Can you work these out from the model? Positions are in its coordinate system, mm. Face numbers are marked on the shaded views. A direction names the side the tool comes from. Coordinates: 2 decimals unless noted, no trailing zeros. Loops run counter-clockwise (first coordinate to the right, second up) from the corner with the lowest first, then second, coordinate; pieces in that order, holes last.
```python
from build123d import *

# Parameters (mm, degrees)
PAD_DEPTH    = 10
SKETCH001_W  = 20
SKETCH001_H  = 50
PAD001_DEPTH = 10
SKETCH002_W  = 20
SKETCH002_H  = 30
PAD002_DEPTH = 20
SKETCH003_W  = 40
SKETCH003_H  = 20
PAD003_DEPTH = 20


with BuildPart() as part:
    # Sketch → Pad (new body)
    with BuildSketch(Plane.XY):
        Polygon((-45, 50), (-45, 0), (15, 0), (15, 20), (45, 20), (45, 50), align=None)
    extrude(amount=PAD_DEPTH)

    # Sketch001 → Pad001 (new body)
    with BuildSketch(Plane.XY.offset(10)):
        with Locations((-35, 25)):
            Rectangle(SKETCH001_W, SKETCH001_H)
    extrude(amount=PAD001_DEPTH)

    # Sketch002 → Pad002 (new body)
    with BuildSketch(Plane.XY.offset(20)):
        with Locations((-35, 35)):
            Rectangle(SKETCH002_W, SKETCH002_H)
    extrude(amount=PAD002_DEPTH)

    # Sketch003 → Pad003 (new body)
    with BuildSketch(Plane.XY.offset(10)):
        with Locations((-5, 40)):
            Rectangle(SKETCH003_W, SKETCH003_H)
    extrude(amount=PAD003_DEPTH)


solid = part.part
```
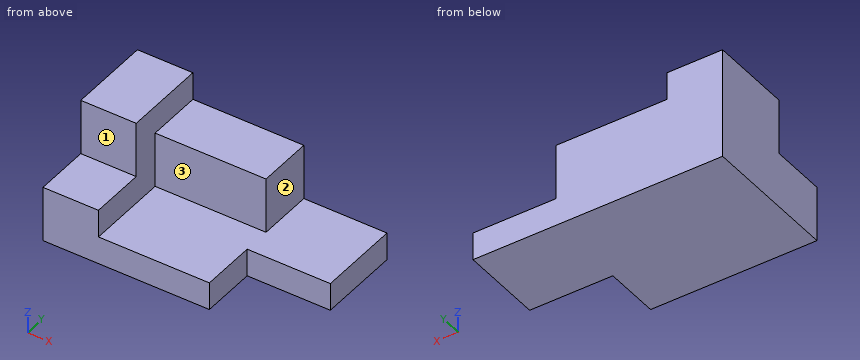
Item 1: On a 3-axis mill with a long thin cutter (end or side, diameter ignored), from which of +Z, -Z, +X, -X, +Y, -Y can I reach the whole of each face in a straight line? I mean the marked faces 1, 2 and 3. Say none if no direction works.
Results are:
face 1: +Z, +X, -X, -Y
face 2: +Z, +X, +Y, -Y
face 3: +Z, +X, -Y
Item 2: Suppose I cut it at D-D, the plane y = 37.5. Please give me the cut outline in (x, z), plus the area to 3 significant figures.
Results are:
outline: (-45, 0) - (45, 0) - (45, 10) - (15, 10) - (15, 30) - (-25, 30) - (-25, 40) - (-45, 40) - close
area: 2,300 mm2
Item 3: Suppose I cut it at B-B, the plane y = 24. Please give me the cut outline in (x, z), plus the area to 3 significant figures.
Results are:
outline: (-45, 0) - (45, 0) - (45, 10) - (-25, 10) - (-25, 40) - (-45, 40) - close
area: 1,500 mm2
Item 4: I'm going to push flat-ended pins straight in: P1, Ø5, axis at x = 7.5, y = 25.5, coming from the +Z side; P2, Ø6, axis at y = 14, z = 24.5, coming from the -X side; P3, Ø15, axis at x = 8.5, y = 37, coming from the +Z side; P4, Ø2, axis at y = 29.5, z = 33.5, coming from the +X side. Where does each tip first touch, or does it pass through?
Results are:
P1: stops at z = 10
P2: passes through
P3: stops at z = 30
P4: stops at x = -25
Item 5: Suppose I cut it at A-A, the plane z = 13. Please give me the cut outline in (x, y), plus the area to 3 significant figures.
Results are:
outline: (-45, 0) - (-25, 0) - (-25, 30) - (15, 30) - (15, 50) - (-45, 50) - close
area: 1,800 mm2
Item 6: I need wall thicknesses on line 1 along Z through (x, y) = (11.5, 24.5); line 2 along Z through (x, y) = (-19.5, 40); line 3 along X through (y, z) = (26.5, 14). Which ranges of each line are inside material? Lowest first, please.
Results are:
line 1: z = 0 to 10
line 2: z = 0 to 30
line 3: x = -45 to -25
Item 7: Suppose I cut it at C-C, the plane x = 17. Please give me the cut outline in (y, z), plus the area to 3 significant figures.
Results are:
outline: (20, 0) - (50, 0) - (50, 10) - (20, 10) - close
area: 300 mm2
